Verification items for the finished model (mm, model axes). Give positions to 0.01 mm unless a question says otherwise; leave off trailing zeros. Loops run counter-clockwise (first coordinate to the right, second up) from the corner with the lowest first, then second, coordinate; pieces in that order, holes last. Notation, with made-up numbers: M -26.5,53.25 L 14.5,53.25 A21 ccw 14.5,59.25 Z; hole C 89.5,78.5 d11. An arc over 180 degrees is marked long. Use CSV: the item, a comma, the result in double quotes.
from build123d import *

# Parameters (mm, degrees)
BOSS_EXTRUDE1_DEPTH = 3.175
FILLET1_R           = 6.35


with BuildPart() as part:
    # Sketch1 → Boss-Extrude1 (new body)
    with BuildSketch(Plane(origin=(0, 0, 0), x_dir=(1, 0, 0), z_dir=(0, 1, 0))):
        Polygon((0, 0), (0, 133.35), (44.45, 133.35), (133.35, 44.45), (133.35, 0), align=None)
    extrude(amount=BOSS_EXTRUDE1_DEPTH)

    # Fillet1
    fillet1_edges = [part.edges().sort_by_distance(p)[0] for p in [
        (0, 1.5875, 0),
        (0, 1.5875, -133.35),
        (44.45, 1.5875, -133.35),
        (133.35, 1.5875, -44.45),
        (133.35, 1.5875, 0),
    ]]
    fillet(fillet1_edges, radius=FILLET1_R)


solid = part.part
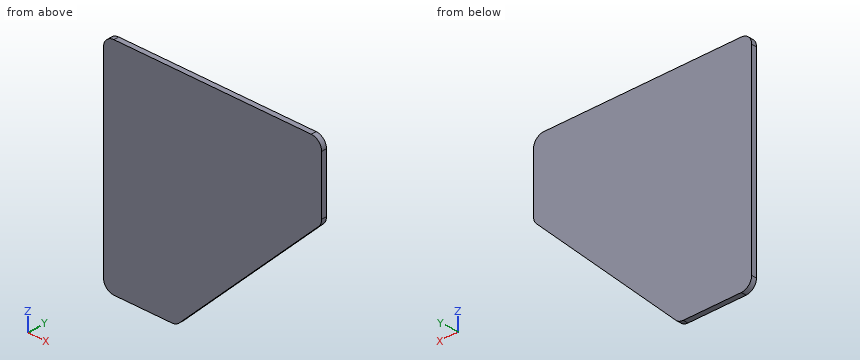
(1) Scan lines: L1, parallel to X at y = 2.95, z = -118.5; L2, parallel to X at y = 1.7, z = -78; L3, parallel to Z at x = 85.5, y = 1.75. Record each from-to range of solid material in increasing order. Write a range as from..to.
Calculated:
L1,"x = 0..59.3"
L2,"x = 0..99.8"
L3,"z = -92.3..0"
(2) Depth check by flat-ended pin: pin 1 Ø1.5 at (y, z) = (2.5, -60.5) entering from +X. Enter the tip coordinate at first touch or a pass-through.
Calculated:
pin 1,"stops at x = 118.05"
(3) Section check A-A on y = 0.55. Record the cut outline in (x, z), plus the area to 3 significant figures.
Calculated:
outline,"M 0,-127 A6.35 ccw 6.35,-133.35 L 41.82,-133.35 A6.35 ccw 46.31,-131.49 L 131.49,-46.31 A6.35 ccw 133.35,-41.82 L 133.35,-6.35 A6.35 ccw 127,0 L 6.35,0 A6.35 ccw 0,-6.35 Z"
area,"13,800 mm²"
(4) Section check C-C on x = 83. Record the cut outline in (y, z) (3 decimals), plus the area to 3 significant figures.
Calculated:
outline,"M 0,-94.8 L 3.175,-94.8 L 3.175,0 L 0,0 Z"
area,"301 mm²"
(5) Section check B-B on z = -116.5. Record the cut outline in (x, y) (3 decimals).
Calculated:
outline,"M 0,0 L 61.3,0 L 61.3,3.175 L 0,3.175 Z"
